from build123d import *

# Parameters (mm, degrees)
SKETCH1_R                = 15.875
SKETCH1_R_2              = 6.5
SKETCH1_R_3              = 0.79375
BOSS_EXTRUDE1_DEPTH      = 5.8
M3_CLEARANCE_HOLE1_D     = 3.2
M3_CLEARANCE_HOLE1_DEPTH = 5.8
M3_CLEARANCE_HOLE1_TIP   = 0.96137699


with BuildPart() as part:
    # Sketch1 → Boss-Extrude1 (new body)
    with BuildSketch(Plane.XY):
        Circle(SKETCH1_R)
        Circle(SKETCH1_R_2, mode=Mode.SUBTRACT)
        with Locations((0, 11.90625)):
            Circle(SKETCH1_R_3, mode=Mode.SUBTRACT)
        with Locations((-11.90625, 0)):
            Circle(SKETCH1_R_3, mode=Mode.SUBTRACT)
        with Locations((0, -11.90625)):
            Circle(SKETCH1_R_3, mode=Mode.SUBTRACT)
        with Locations((11.90625, 0)):
            Circle(SKETCH1_R_3, mode=Mode.SUBTRACT)
    extrude(amount=BOSS_EXTRUDE1_DEPTH)

    # M3 Clearance Hole1
    with Locations(Plane.XY.offset(5.8)):
        with Locations((-8.418990114, 8.418990114), (8.418990114, 8.418990114), (8.418990114, -8.418990114), (-8.418990114, -8.418990114)):
            Hole(M3_CLEARANCE_HOLE1_D / 2, depth=M3_CLEARANCE_HOLE1_DEPTH)
            with Locations((0, 0, -(M3_CLEARANCE_HOLE1_DEPTH + M3_CLEARANCE_HOLE1_TIP / 2))):  # 118° drill point
                Cone(0, M3_CLEARANCE_HOLE1_D / 2, M3_CLEARANCE_HOLE1_TIP, mode=Mode.SUBTRACT)


solid = part.part
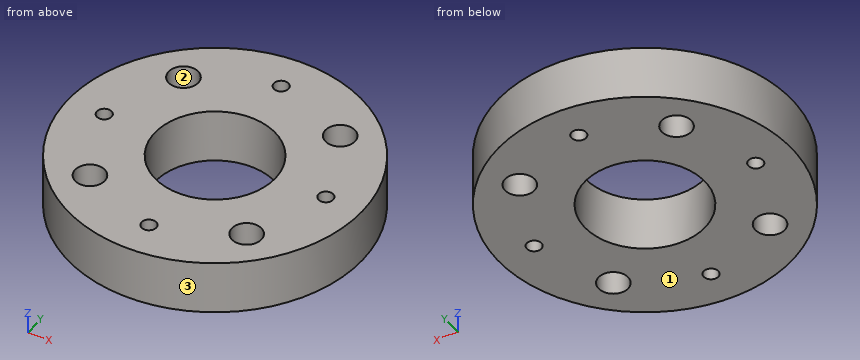
Check sheet for the modelled part. Datum: model origin and axes. Units: mm. Face numbers are marked on the shaded views. Round coordinates to 2 decimals unless told otherwise and drop trailing zeros. Order: outer loops, then holes, each group sorted by start corner. A loop starts at its lowest first (then second) coordinate and runs counter-clockwise, first axis right, second up.
(1) Go/stop test with flat-tipped pins: P1, Ø3, axis at x = 10.5, z = 3.5, coming from the -Y side; P2, Ø1, axis at y = -2.5, z = 2.5, coming from the -X side; P3, Ø1.5, axis at x = -8, z = 3.5, coming from the +Y side; P4, Ø1.9, axis at x = 8.42, y = -8.42, coming from the -Z side. Record where each tip stops, or that it passes through.
(2) Draft check along X on the marked faces 1, 2 and 3. Enter one of: pulls with the +X half, pulls with the -X half, needs draft (parallel to the pull), parting line crosses it, or undercut.
(3) Cross-section at C-C, the plane x = 8.5. Enter the section's corners in (y, z), and give its area (3 significant figures).
(4) Scan lines: probe 1 along Y at (x, z) = (9, 1); probe 2 along Y at (x, z) = (0, 3.8) (1 decimal); probe 3 along Y at (x, z) = (8, 1.7). Record each from-to range of solid material in increasing order.
(5) Cross-section at A-A, the plane x = 0. Enter the section's corners in (y, z) (1 decimal).
(6) Cross-section at D-D, the plane y = 6. Enter the section's corners in (x, z).
Check sheet entries:
1. P1: stops at y = -13.08
1. P2: stops at x = -15.75
1. P3: stops at y = 14.12
1. P4: passes through
2. face 1: needs draft
2. face 2: undercut
2. face 3: parting line crosses it
3. outline: (-13.41, 0) - (-10.02, 0) - (-10.02, 5.8) - (-13.41, 5.8) - close; (-6.82, 0) - (6.82, 0) - (6.82, 5.8) - (-6.82, 5.8) - close; (10.02, 0) - (13.41, 0) - (13.41, 5.8) - (10.02, 5.8) - close
3. area: 118 mm2
4. probe 1: y = -13.08 to -9.91, -6.93 to 6.93, 9.91 to 13.08
4. probe 2: y = -15.9 to -12.7, -11.1 to -6.5, 6.5 to 11.1, 12.7 to 15.9
4. probe 3: y = -13.71 to -9.96, -6.87 to 6.87, 9.96 to 13.71
5. outline: (-15.9, 0) - (-12.7, 0) - (-12.7, 5.8) - (-15.9, 5.8) - close; (-11.1, 0) - (-6.5, 0) - (-6.5, 5.8) - (-11.1, 5.8) - close; (6.5, 0) - (11.1, 0) - (11.1, 5.8) - (6.5, 5.8) - close; (12.7, 0) - (15.9, 0) - (15.9, 5.8) - (12.7, 5.8) - close
6. outline: (-14.7, 0) - (-2.5, 0) - (-2.5, 5.8) - (-14.7, 5.8) - close; (2.5, 0) - (14.7, 0) - (14.7, 5.8) - (2.5, 5.8) - close
